Check sheet for the modelled part. Datum: model origin and axes. Units: mm. Round coordinates to 2 decimals unless told otherwise and drop trailing zeros. Loops run counter-clockwise (first coordinate to the right, second up) from the corner with the lowest first, then second, coordinate; pieces in that order, holes last. Notation, with made-up numbers: M 64,-21.75 L 71,-21.75 A21 cw 71,-12.75 Z; hole C 73,67 d6. An arc over 180 degrees is marked long. Write item = value, one per line. Start each with the question number.
(1) Scan lines: L1, parallel to Y at x = 396, z = 4.75; L2, parallel to X at y = 292, z = 1.5; L3, parallel to Y at x = 422, z = 1.05. Record each from-to range of solid material in increasing order. Write a range as from..to.
(2) Cross-section at C-C on x = 409. Record the boundary of the cut face in (y, z).
(3) Cross-section at B-B on y = 295.5. Record the boundary of the cut face in (x, z), plus the area to 3 significant figures.
(4) Go/stop test with flat-tipped pins: P1, Ø3, axis at y = 323.5, z = 4, coming from the -X side; P2, Ø6, axis at x = 435, y = 373, coming from the -Z side; P3, Ø3, axis at x = 387.5, z = 2, coming from the -Y side. Record where each tip stops, or that it passes through.
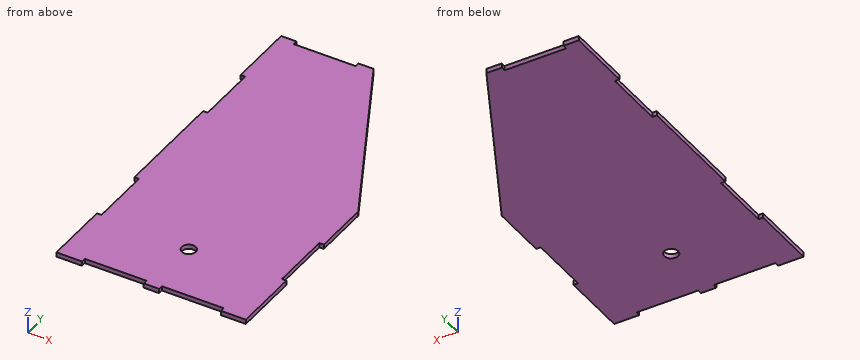
from build123d import *

# Parameters (mm, degrees)
BOSS_EXTRUDE3_DEPTH     = 5.588
SKETCH2_W               = 76.2
SKETCH2_H               = 5.588
SKETCH2_W_2             = 5.588
SKETCH2_H_2             = 76.2
CUT_EXTRUDE1_DEPTH      = 850.582717671
CUT_EXTRUDE3_DEPTH      = 850.582717671
CUT_EXTRUDE3_DEPTH_BACK = 850.582717671
SKETCH3_R               = 8.636


with BuildPart() as part:
    # Sketch1 → Boss-Extrude3 (new body)
    with BuildSketch(Plane.XY):
        Polygon((435.519883673, 642.86985555), (555.407883673, 414.26985555), (555.407883673, 185.66985555), (321.219883673, 185.66985555), (321.219883673, 642.86985555), align=None)
    extrude(amount=BOSS_EXTRUDE3_DEPTH)

    # Sketch2 → Cut-Extrude1 (cut, through all)
    with BuildSketch(Plane.XY.offset(5.588)):
        with Locations((378.369883673, 640.07585555)):
            Rectangle(SKETCH2_W, SKETCH2_H)
        with Locations((324.013883673, 522.21985555)):
            Rectangle(SKETCH2_W_2, SKETCH2_H_2)
        with Locations((324.013883673, 306.31985555)):
            Rectangle(SKETCH2_W_2, SKETCH2_H_2)
        with Locations((391.069883673, 188.46385555)):
            Rectangle(SKETCH2_W, SKETCH2_H)
        with Locations((486.319883673, 188.46385555)):
            Rectangle(SKETCH2_W, SKETCH2_H)
        with Locations((552.613883673, 306.31985555)):
            Rectangle(SKETCH2_W_2, SKETCH2_H_2)
    extrude(amount=-CUT_EXTRUDE1_DEPTH, mode=Mode.SUBTRACT)

    # Sketch3 → Cut-Extrude3 (cut, two sides: drawn at the far end of the back side and taken through both)
    with BuildSketch(Plane.XY.offset(-CUT_EXTRUDE3_DEPTH_BACK)):
        with Locations((437.932883673, 262.989065336)):
            Circle(SKETCH3_R)
    extrude(amount=CUT_EXTRUDE3_DEPTH + CUT_EXTRUDE3_DEPTH_BACK, mode=Mode.SUBTRACT)


solid = part.part
Result:
q1.L1 = 191.26..637.28
q1.L2 = 326.81..549.82
q1.L3 = 191.26..642.87
q2.outline = M 191.26,0 L 637.28,0 L 637.28,5.59 L 191.26,5.59 Z
q3.outline = M 326.81,0 L 549.82,0 L 549.82,5.59 L 326.81,5.59 Z
q3.area = 1,250 mm^2
q4.P1 = 326.81
q4.P2 = 0
q4.P3 = 191.26
